Verification items for this drawing (mm, ordinates from the low corner). Round coordinates to 2 decimals unless told otherwise and drop trailing zeros. Loops run counter-clockwise (first coordinate to the right, second up) from the corner with the lowest first, then second, coordinate; pieces in that order, holes last. Notation, with made-up numbers: (26.25, 81.5) - (44.25, 81.5) arc R13 cw to (44.25, 96.5) - close; hole circle Ø1 at (70, 45.25). An arc over 180 degrees is marked (long way). Use a Markdown table: item, result. Add a question column.
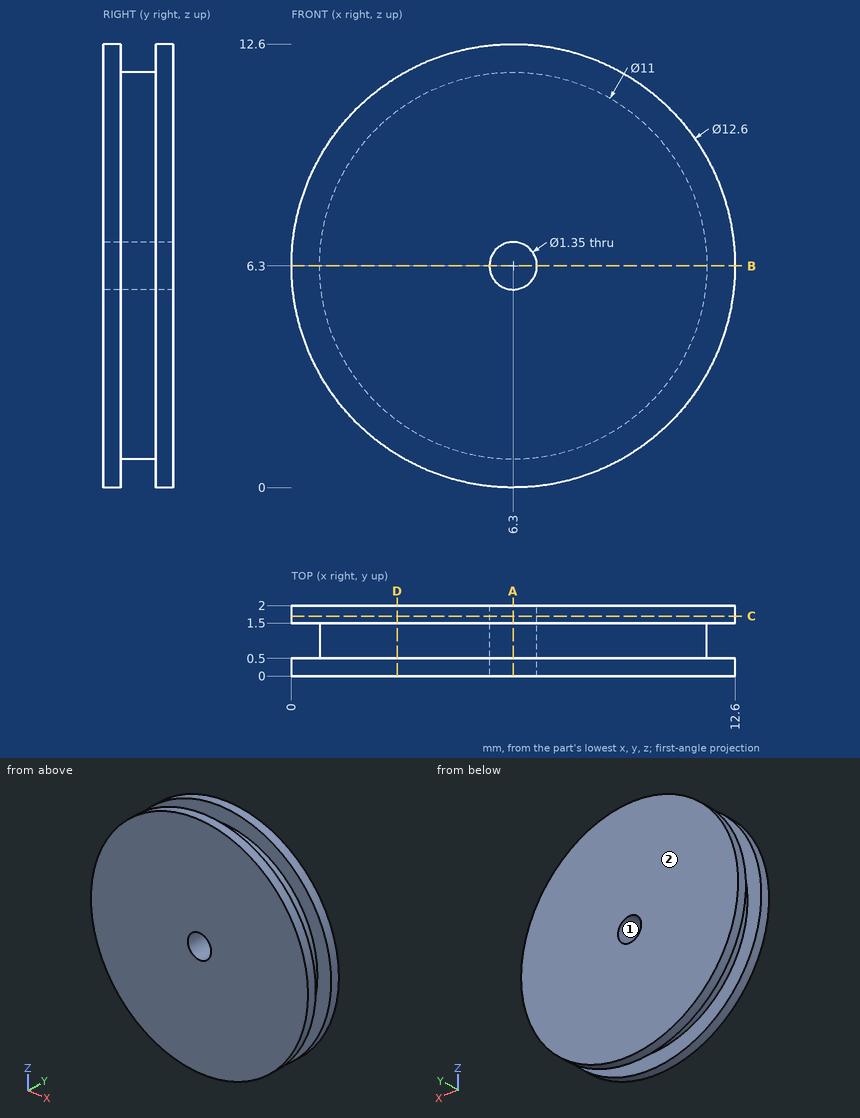
Q1. Thickness scan on line 1 along Z through (x, y) = (6.3, 1.2) (3 decimals); line 2 along X through (y, z) = (0.45, 6.5); line 3 along Z through (x, y) = (9.25, 0.7). Record the ranges inside material, lowest first.
Q2. Section check A-A on x = 6.3. Record the cut outline in (y, z) (3 decimals).
Q3. Section check D-D on x = 3. Record the cut outline in (y, z), plus the area to 3 significant figures.
Q4. Section check C-C on y = 1.7. Record the cut outline in (x, z) (3 decimals), plus the area to 3 significant figures.
Q5. Release check for a two-part mould opening along X. For the marked faces 1 and 2 record: +X half, -X half, draft (parallel to the pull), parting line (faces both ways), or undercut.
Q6. Section check B-B on z = 6.3. Record the cut outline in (x, y) (3 decimals), plus the area to 3 significant figures.
Determined:
| question | item | result |
|---|---|---|
| 1 | line 1 | z = 0.8 to 5.625, 6.975 to 11.8 |
| 1 | line 2 | x = 0 to 5.66, 6.94 to 12.6 |
| 1 | line 3 | z = 1.66 to 10.94 |
| 2 | outline | (0, 0) - (0.5, 0) - (0.5, 0.8) - (1.5, 0.8) - (1.5, 0) - (2, 0) - (2, 5.625) - (0, 5.625) - close; (0, 6.975) - (2, 6.975) - (2, 12.6) - (1.5, 12.6) - (1.5, 11.8) - (0.5, 11.8) - (0.5, 12.6) - (0, 12.6) - close |
| 3 | outline | (0, 0.93) - (0.5, 0.93) - (0.5, 1.9) - (1.5, 1.9) - (1.5, 0.93) - (2, 0.93) - (2, 11.67) - (1.5, 11.67) - (1.5, 10.7) - (0.5, 10.7) - (0.5, 11.67) - (0, 11.67) - close |
| 3 | area | 19.5 mm² |
| 4 | outline | circle Ø12.6 at (6.3, 6.3); hole circle Ø1.35 at (6.3, 6.3) |
| 4 | area | 123 mm² |
| 5 | face 1 | undercut |
| 5 | face 2 | draft |
| 6 | outline | (0, 0) - (5.625, 0) - (5.625, 2) - (0, 2) - (0, 1.5) - (0.8, 1.5) - (0.8, 0.5) - (0, 0.5) - close; (6.975, 0) - (12.6, 0) - (12.6, 0.5) - (11.8, 0.5) - (11.8, 1.5) - (12.6, 1.5) - (12.6, 2) - (6.975, 2) - close |
| 6 | area | 20.9 mm² |
